from build123d import *

# Parameters (mm, degrees)
SKETCH3_W           = 20
SKETCH3_H           = 50
BOSS_EXTRUDE2_DEPTH = 2
SKETCH4_R           = 3
SKETCH4_R_2         = 2
BOSS_EXTRUDE3_DEPTH = 50


with BuildPart() as part:
    # Sketch3 → Boss-Extrude2 (new body)
    with BuildSketch(Plane.XY):
        Rectangle(SKETCH3_W, SKETCH3_H)
    extrude(amount=BOSS_EXTRUDE2_DEPTH)

    # Sketch4 → Boss-Extrude3 (add)
    with BuildSketch(Plane(origin=(0, 25, 0), x_dir=(1, 0, 0), z_dir=(0, 1, 0))):
        with Locations((12.5, -1.5)):
            Circle(SKETCH4_R)
        with Locations((12.5, -1.5)):
            Circle(SKETCH4_R_2, mode=Mode.SUBTRACT)
    extrude(amount=-BOSS_EXTRUDE3_DEPTH)


solid = part.part
The listing builds one solid part. Answer for the finished solid, in the listing's coordinates (mm). A direction names the side the tool comes from. Round coordinates to 2 decimals unless told otherwise and drop trailing zeros. Order: outer loops, then holes, each group sorted by start corner. A loop starts at its lowest first (then second) coordinate and runs counter-clockwise, first axis right, second up. Notation, with made-up numbers: M 50.25,70.25 L 105.25,70.25 A7 ccw 105.25,82.25 Z; hole C 75.5,78 d7. An arc over 180 degrees is marked long. Answer in a Markdown table with one row per item. Add a question column.
1) The part is cut by section D-D on x = 8.5. Determine the outline of the cut face in (y, z), plus the area to 3 significant figures.
2) The part is cut by section C-C on y = -12. Determine the outline of the cut face in (x, z), plus the area to 3 significant figures.
3) Which of the six approach directions +Z, -Z, +X, -X, +Y, -Y give full straight-line access (tool end or side, diameter ignored) to faces 1 (the face through (-10, 0, 1)), 2 (the face through (0, 0, 2))?
4) The part is cut by section A-A on z = 1.5. Determine the outline of the cut face in (x, y).
5) The part is cut by section B-B on x = 12.5. Determine the outline of the cut face in (y, z).
6) Flat-ended cylindrical pins translate along their axes: pin 1 Ø2 at (x, y) = (3.5, -7) entering from +Z; pin 2 Ø10 at (x, y) = (-2, -0.5) entering from -Z; pin 3 Ø1.5 at (x, z) = (8.5, 3.5) entering from +Y. Find the tip coordinate at first contact, or state that the pin passes through.
7) Determine the mould class of faces 3 (the face through (10.9, 0.4, 2.7)), 4 (the face through (15.43, 0.35, 2.15)), 5 (the face through (0, 0, 0)), 6 (the face through (4, -25, 1)) for opening direction Z: pulls with the +Z half, pulls with the -Z half, needs draft (parallel to the pull), parting line crosses it, or undercut.
8) Consider line 1 along Z through (x, y) = (12.5, 7.5); line 2 along X through (y, z) = (9.5, 1.5); line 3 along Z through (x, y) = (1.5, 3). Determine where each line is inside the solid, lowest interval first. Write a range as from..to.
Findings below:
| question | item | result |
|---|---|---|
| 1 | outline | M -25,0 L 25,0 L 25,2 L -25,2 Z |
| 1 | area | 100 mm² |
| 2 | outline | M -10,0 L 9.9,0 A3 ccw long 9.54,2 L -10,2 Z; hole C 12.5,1.5 d4 |
| 2 | area | 54.9 mm² |
| 3 | face 1 | +Z, -Z, -X, +Y, -Y |
| 3 | face 2 | +Z, -X, +Y, -Y |
| 4 | outline | M -10,-25 L 10.5,-25 L 10.5,25 L -10,25 Z; M 14.5,-25 L 15.5,-25 L 15.5,25 L 14.5,25 Z |
| 5 | outline | M -25,-1.5 L 25,-1.5 L 25,-0.5 L -25,-0.5 Z; M -25,3.5 L 25,3.5 L 25,4.5 L -25,4.5 Z |
| 6 | pin 1 | stops at z = 2 |
| 6 | pin 2 | stops at z = 0 |
| 6 | pin 3 | passes through |
| 7 | face 3 | undercut |
| 7 | face 4 | parting line crosses it |
| 7 | face 5 | pulls with the -Z half |
| 7 | face 6 | needs draft |
| 8 | line 1 | z = -1.5..-0.5, 3.5..4.5 |
| 8 | line 2 | x = -10..10.5, 14.5..15.5 |
| 8 | line 3 | z = 0..2 |
